Here's how the part is built. I have some questions about the finished solid (model axes, mm). Coordinates: 2 decimals unless noted, no trailing zeros. Write each loop counter-clockwise with the first axis right and the second up, starting at its lowest first coordinate (ties: lowest second). Pieces come first, ordered by that corner, then holes. Notation, with made-up numbers: (77.5, 38.5) -> (95.5, 38.5) arc R21 ccw to (95.5, 54.5) -> close; hole circle Ø11 at (-33, 20). An arc over 180 degrees is marked (long way). Use a Markdown table: item, result. Add a question column.
Autodesk Fusion 360 part; units mm, degrees
sketch "スケッチ1" plane through (0, 0, 0) normal (0, 0, 1) x (1, 0, 0)
  line L0 (2.5, 186) -> (-92.5, 186)
  line L1 (-92.5, 186) -> (-92.5, -186)
  line L2 (-92.5, -186) -> (2.5, -186)
  line L3 (92.5, -50) -> (92.5, 180)
  line L4 (89.5161, 180) -> (-92.5, -186) construction
  line L5 (-92.5, 186) -> (53.8847, -108.352) construction
  line L6 (2.5, 186) -> (2.5, 180)
  line L7 (2.5, 180) -> (92.5, 180)
  line L8 (-92.5, -186) -> (2.5, -186) construction
  line L9 (92.5, -50) -> (2.5, -186)
  dimension "d2" = 372
  dimension "d5" = 95
extrude "押し出し1" add sketch "スケッチ1" along normal blind 6
chamfer "面取り1" distance 30 angle 45 2 edges at (-92.5, -186, 3) (-92.5, 186, 3)
sketch "スケッチ2" plane through (0, 0, 6) normal (0, 0, 1) x (-1, 0, 0)
  line L0 (62.5, -186) -> (92.5, -156)
  line L1 (92.5, -156) -> (92.5, 156)
  line L2 (92.5, 156) -> (62.5, 186)
  line L3 (62.5, 186) -> (-2.5, 186)
  line L4 (-2.5, 186) -> (-92.5, 50)
  line L5 (-92.5, 50) -> (-92.5, -180)
  line L6 (-92.5, -180) -> (-2.5, -180)
  line L7 (-2.5, -180) -> (-2.5, -186)
  line L8 (-2.5, -186) -> (62.5, -186)
  line L9 (-92.5, -180) -> (-52.5, -180) construction
  line L10 (-52.5, -180) -> (-52.5, -135) construction
  line L11 (-52.5, -135) -> (-92.5, -135) construction
  line L12 (-92.5, -135) -> (-92.5, -180) construction
  line L13 (-52.5, -135) -> (-52.5, -75) construction
  line L14 (-52.5, -75) -> (-52.5, -15) construction
  point P0 (-52.5, -135)
  point P1 (-52.5, -75)
  point P2 (-52.5, -15)
  dimension "d10" = 40
  dimension "d11" = 45
  dimension "d12" = 60
  dimension "d13" = 60
hole "穴1" at (52.5, 135, 6) at (52.5, 75, 6) at (52.5, 15, 6) at (52.5, 15, 6) direction (0, 0, -1) diameter 18 end through all
equation "d5 = 30 mm + 65 mm"
Q1. Suppose I cut it at C-C, the plane x = 52.5. Write out the boundary of the cut face in (y, z).
Q2. Will this pin go through, and if not, where does the flat tip stop? pin 1 (3 mm diameter, centred on y = -142.5, z = 5, fed in from +X).
Q3. Suppose I cut it at A-A, the plane y = 135. Write out the boundary of the cut face in (x, z).
Q4. Suppose I cut it at B-B, the plane z = 2.3. Write out the boundary of the cut face in (x, y).
Q5. Suppose I cut it at D-D, the plane x = 34. Write out the boundary of the cut face in (y, z).
Q6. Thinking about a two-plate mould opening in X: for faces 1 (the cylindrical face through (49.797, 6.416, 2.958)), 2 (the flat face through (-1, 3, 6)), 3 (the cylindrical face through (49.797, 66.416, 2.958)), 4 (the flat face through (-77.3, 171.2, 3)), which applies, released by +X, released by -X, zero draft, split by the parting line, or undercut?
Q7. Please list where these lines run through material, in increasing order: line 1 (Y direction, x = 52.5, z = 4.7); line 2 (X direction, y = 15, z = 4.35); line 3 (Y direction, x = 10.5, z = 2.9).
Answer key:
| question | item | result |
|---|---|---|
| 1 | outline | (-110.44, 0) -> (6, 0) -> (6, 6) -> (-110.44, 6) -> close; (24, 0) -> (66, 0) -> (66, 6) -> (24, 6) -> close; (84, 0) -> (126, 0) -> (126, 6) -> (84, 6) -> close; (144, 0) -> (180, 0) -> (180, 6) -> (144, 6) -> close |
| 2 | pin 1 | stops at x = 32.28 |
| 3 | outline | (-92.5, 0) -> (43.5, 0) -> (43.5, 6) -> (-92.5, 6) -> close; (61.5, 0) -> (92.5, 0) -> (92.5, 6) -> (61.5, 6) -> close |
| 4 | outline | (-92.5, -156) -> (-62.5, -186) -> (2.5, -186) -> (92.5, -50) -> (92.5, 180) -> (2.5, 180) -> (2.5, 186) -> (-62.5, 186) -> (-92.5, 156) -> close; hole circle Ø18 at (52.5, 15); hole circle Ø18 at (52.5, 75); hole circle Ø18 at (52.5, 135) |
| 5 | outline | (-138.4, 0) -> (180, 0) -> (180, 6) -> (-138.4, 6) -> close |
| 6 | face 1 | undercut |
| 6 | face 2 | zero draft |
| 6 | face 3 | undercut |
| 6 | face 4 | released by -X |
| 7 | line 1 | y = -110.44 to 6, 24 to 66, 84 to 126, 144 to 180 |
| 7 | line 2 | x = -92.5 to 43.5, 61.5 to 92.5 |
| 7 | line 3 | y = -173.91 to 180 |
